Here's how the part is built. I have some questions about the finished solid (model axes, mm). Face numbers are marked on the shaded views. A direction names the side the tool comes from. Round coordinates to 2 decimals unless told otherwise and drop trailing zeros. Loops run counter-clockwise (first coordinate to the right, second up) from the corner with the lowest first, then second, coordinate; pieces in that order, holes last. Notation, with made-up numbers: M 47,38 L 51,38 A27 ccw 51,68 Z; hole C 61.25,46.25 d7. An arc over 180 degrees is marked long. Use a Markdown table: item, result.
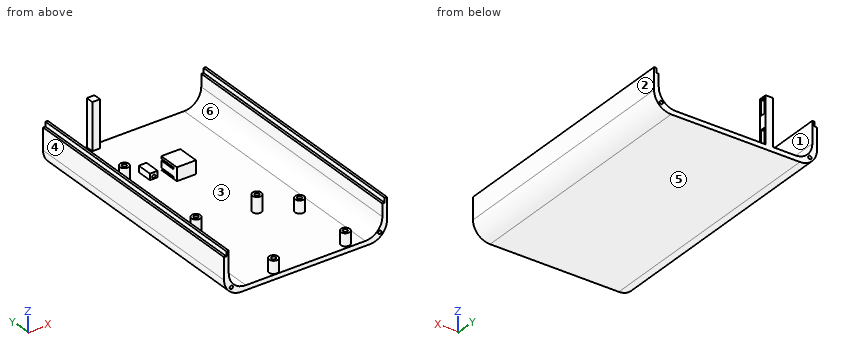
from build123d import *

# Parameters (mm, degrees)
EXTRUDE_1_DEPTH       = 162.5
SKETCH_2_W            = 1.5
SKETCH_2_H            = 162.5
EXTRUDE_2_DEPTH       = 3
SKETCH_2_4_W          = 1.5
SKETCH_2_4_H          = 162.5
CUT_EXTRUDE_2_DEPTH   = 3
SKETCH_3_R            = 1.05
CUT_EXTRUDE_3_DEPTH   = 4
CUT_EXTRUDE_START     = -4
SKETCH_4_R            = 1.05
CUT_EXTRUDE_4_DEPTH   = 4
SKETCH_6_R            = 2.9
SKETCH_6_R_2          = 1.4
EXTRUDE_1_2_DEPTH     = 10
SKETCH_7_R            = 2.9
SKETCH_7_R_2          = 1.4
EXTRUDE_2_2_DEPTH     = 8
EXTRUDE_4_DEPTH       = 8.5
CUT_EXTRUDE_6_REACH   = 176.56
SKETCH_13_W           = 1.2
SKETCH_13_H           = 11
EXTRUDE_START         = 1.4
EXTRUDE_5_OUTLINE_W   = 0.5
EXTRUDE_5_OUTLINE_H   = 1.8
EXTRUDE_5_DEPTH       = 4.4
EXTRUDE_5_2_OUTLINE_W = 5
EXTRUDE_5_2_OUTLINE_H = 10
EXTRUDE_5_2_DEPTH     = 4
EXTRUDE_START_2       = 116
EXTRUDE_6_OUTLINE_R   = 1.05
EXTRUDE_6_DEPTH       = 10
EXTRUDE_START_3       = 157.5
EXTRUDE_6_2_OUTLINE_W = 5
EXTRUDE_6_2_OUTLINE_H = 30
EXTRUDE_6_2_DEPTH     = 5
EXTRUDE_START_4       = -7.5
EXTRUDE_7_OUTLINE_W   = 2.9
EXTRUDE_7_OUTLINE_H   = 2.85
EXTRUDE_7_DEPTH       = 9.65
EXTRUDE_START_5       = 10.85
EXTRUDE_7_2_OUTLINE_W = 2.9
EXTRUDE_7_2_OUTLINE_H = 2.85
EXTRUDE_7_2_DEPTH     = 9.65
EXTRUDE_START_6       = -1.5
EXTRUDE_7_3_OUTLINE_W = 8.3
EXTRUDE_7_3_OUTLINE_H = 11.95
EXTRUDE_7_3_DEPTH     = 1.5


# Read off the part's stored shape, not the designer's step: 凸台-拉伸5, 凸台-拉伸6, 凸台-拉伸7
with BuildPart() as part:
    # 草图1 → Extrude 1 (new body)
    with BuildSketch(Plane(origin=(0, 0, 0), x_dir=(1, 0, 0), z_dir=(0, 1, 0))):
        with BuildLine():
            Line((-3, 0), (-3, 14))
            ThreePointArc((-3, 14), (0.221825407, 21.778174593), (8, 25))
            Line((8, 25), (91, 25))
            ThreePointArc((91, 25), (98.778174593, 21.778174593), (102, 14))
            Line((102, 14), (102, 0))
            Line((102, 0), (99, 0))
            Line((99, 0), (99, 11))
            ThreePointArc((99, 11), (95.778174593, 18.778174593), (88, 22))
            Line((88, 22), (11, 22))
            ThreePointArc((11, 22), (3.221825407, 18.778174593), (0, 11))
            Line((0, 11), (0, 0))
            Line((0, 0), (-3, 0))
        make_face()
    extrude(amount=EXTRUDE_1_DEPTH)

    # 草图2 → Extrude 2 (add)
    with BuildSketch(Plane.XY):
        with Locations((-0.75, 81.25)):
            Rectangle(SKETCH_2_W, SKETCH_2_H)
    extrude(amount=EXTRUDE_2_DEPTH)

    # 草图2<4> → 切除-拉伸2 (cut)
    with BuildSketch(Plane.XY):
        with Locations((99.75, 81.25)):
            Rectangle(SKETCH_2_4_W, SKETCH_2_4_H)
    extrude(amount=-CUT_EXTRUDE_2_DEPTH, mode=Mode.SUBTRACT)

    # 草图3 → 切除-拉伸3 (cut)
    with BuildSketch(Plane(origin=(0, 162.5, 0), x_dir=(1, 0, 0), z_dir=(0, 1, 0))):
        with Locations(Location((1.61916848, 20, 0), (0, 0, 270))):
            Circle(SKETCH_3_R)
        with Locations(Location((97.38083152, 20, 0), (0, 0, 270))):
            Circle(SKETCH_3_R)
    extrude(amount=-CUT_EXTRUDE_3_DEPTH, mode=Mode.SUBTRACT)

    # 草图4 → 切除-拉伸4 (cut)
    with BuildSketch(Plane.XZ.offset(CUT_EXTRUDE_START)):
        with Locations(Location((1.61916848, -20, 0), (0, 0, 90))):
            Circle(SKETCH_4_R)
        with Locations(Location((97.38083152, -20, 0), (0, 0, 90))):
            Circle(SKETCH_4_R)
    extrude(amount=CUT_EXTRUDE_4_DEPTH, mode=Mode.SUBTRACT)

    # 草图6 → Extrude 1 2 (add)
    # profile 1 of 3: a face of its own
    with BuildSketch(Plane.XY.offset(-22)):
        with Locations((20.69, 122.5)):
            Circle(SKETCH_6_R)
        with Locations((20.69, 122.5)):
            Circle(SKETCH_6_R_2, mode=Mode.SUBTRACT)
    # profile 2 of 3: a face of its own
    with BuildSketch(Plane.XY.offset(-22)):
        with Locations((20.69, 58.19)):
            Circle(SKETCH_6_R)
        with Locations((20.69, 58.19)):
            Circle(SKETCH_6_R_2, mode=Mode.SUBTRACT)
    # profile 3 of 3: a face of its own
    with BuildSketch(Plane.XY.offset(-22)):
        with Locations((60, 58.19)):
            Circle(SKETCH_6_R)
        with Locations((60, 58.19)):
            Circle(SKETCH_6_R_2, mode=Mode.SUBTRACT)
    extrude(amount=EXTRUDE_1_2_DEPTH)

    # 草图7 → Extrude 2 2 (add)
    # profile 1 of 3: a face of its own
    with BuildSketch(Plane.XY.offset(-22)):
        with Locations((78, 4)):
            Circle(SKETCH_7_R)
        with Locations((78, 4)):
            Circle(SKETCH_7_R_2, mode=Mode.SUBTRACT)
    # profile 2 of 3: a face of its own
    with BuildSketch(Plane.XY.offset(-22)):
        with Locations((31.2, 3.2)):
            Circle(SKETCH_7_R)
        with Locations((31.2, 3.2)):
            Circle(SKETCH_7_R_2, mode=Mode.SUBTRACT)
    # profile 3 of 3: a face of its own
    with BuildSketch(Plane.XY.offset(-22)):
        with Locations((78, 45)):
            Circle(SKETCH_7_R)
        with Locations((78, 45)):
            Circle(SKETCH_7_R_2, mode=Mode.SUBTRACT)
    extrude(amount=EXTRUDE_2_2_DEPTH)

    # 草图12 → 凸台-拉伸4 (add)
    with BuildSketch(Plane.XY.offset(-22)):
        Polygon((45.35, 120.9), (45.35, 108.95), (53.65, 108.95), (53.65, 120.9), (55.65, 120.9), (55.65, 106.9), (43.35, 106.9), (43.35, 120.9), align=None)
    extrude(amount=EXTRUDE_4_DEPTH)

    # 切除-拉伸6: up to this face of the body (flat: up to its plane)
    cut_extrude_6_end = Plane(part.part.faces().sort_by_distance((43.35, 113.9, -17.75))[0])
    # 草图13 → 切除-拉伸6 (cut, up to the picked face)
    with BuildSketch(Plane(origin=(55.65, 0, 0), x_dir=(0, 0, -1), z_dir=(1, 0, 0)), mode=Mode.PRIVATE) as cut_extrude_6_sk1:
        with Locations((15.6, 115.4)):
            Rectangle(SKETCH_13_W, SKETCH_13_H)
    cut_extrude_6_tool1 = split(extrude(cut_extrude_6_sk1.sketch, amount=-CUT_EXTRUDE_6_REACH, mode=Mode.PRIVATE), bisect_by=cut_extrude_6_end, keep=Keep.BOTH, mode=Mode.PRIVATE)
    # 草图13 → 切除-拉伸6 (cut, up to the picked face)
    with BuildSketch(Plane(origin=(55.65, 0, 0), x_dir=(0, 0, -1), z_dir=(1, 0, 0)), mode=Mode.PRIVATE) as cut_extrude_6_sk2:
        with Locations((21.2, 115.4)):
            Rectangle(SKETCH_13_W, SKETCH_13_H)
    cut_extrude_6_tool2 = split(extrude(cut_extrude_6_sk2.sketch, amount=-CUT_EXTRUDE_6_REACH, mode=Mode.PRIVATE), bisect_by=cut_extrude_6_end, keep=Keep.BOTH, mode=Mode.PRIVATE)
    add(cut_extrude_6_tool1.solids().sort_by(Axis((55.65, 115.4, -15.6), (-1, 0, 0)))[0], mode=Mode.SUBTRACT)
    add(cut_extrude_6_tool2.solids().sort_by(Axis((55.65, 115.4, -21.2), (-1, 0, 0)))[0], mode=Mode.SUBTRACT)

    # 凸台-拉伸5 outline → 凸台-拉伸5 (cut)
    with BuildSketch(Plane.XY.offset(-22).offset(EXTRUDE_START)):
        with Locations((53.9, 118.25)):
            Rectangle(EXTRUDE_5_OUTLINE_W, EXTRUDE_5_OUTLINE_H)
        with Locations((45.1, 118.25)):
            Rectangle(EXTRUDE_5_OUTLINE_W, EXTRUDE_5_OUTLINE_H)
    extrude(amount=EXTRUDE_5_DEPTH, mode=Mode.SUBTRACT)

    # Extrude 5 2 outline → Extrude 5 2 (add)
    with BuildSketch(Plane.XY.offset(-22)):
        with Locations((35, 121)):
            Rectangle(EXTRUDE_5_2_OUTLINE_W, EXTRUDE_5_2_OUTLINE_H)
    extrude(amount=EXTRUDE_5_2_DEPTH)

    # 凸台-拉伸6 outline → 凸台-拉伸6 (cut)
    with BuildSketch(Plane(origin=(0, 0, 0), x_dir=(1, 0, 0), z_dir=(0, 1, 0)).offset(EXTRUDE_START_2)):
        with Locations((35, 20.5)):
            Circle(EXTRUDE_6_OUTLINE_R)
    extrude(amount=EXTRUDE_6_DEPTH, mode=Mode.SUBTRACT)

    # Extrude 6 2 outline → Extrude 6 2 (add)
    with BuildSketch(Plane(origin=(0, 0, 0), x_dir=(1, 0, 0), z_dir=(0, 1, 0)).offset(EXTRUDE_START_3)):
        with Locations((27.7, 7)):
            Rectangle(EXTRUDE_6_2_OUTLINE_W, EXTRUDE_6_2_OUTLINE_H)
    extrude(amount=EXTRUDE_6_2_DEPTH)

    # 凸台-拉伸7 outline → 凸台-拉伸7 (cut)
    with BuildSketch(Plane.XY.offset(-13.5).offset(EXTRUDE_START_4)):
        with Locations((28.75, 160.075)):
            Rectangle(EXTRUDE_7_OUTLINE_W, EXTRUDE_7_OUTLINE_H)
    extrude(amount=EXTRUDE_7_DEPTH, mode=Mode.SUBTRACT)

    # Extrude 7 2 outline → Extrude 7 2 (cut)
    with BuildSketch(Plane.XY.offset(-13.5).offset(EXTRUDE_START_5)):
        with Locations((28.75, 160.075)):
            Rectangle(EXTRUDE_7_2_OUTLINE_W, EXTRUDE_7_2_OUTLINE_H)
    extrude(amount=EXTRUDE_7_2_DEPTH, mode=Mode.SUBTRACT)

    # Extrude 7 3 outline → Extrude 7 3 (add)
    with BuildSketch(Plane.XY.offset(-13.5).offset(EXTRUDE_START_6)):
        with Locations((49.5, 114.925)):
            Rectangle(EXTRUDE_7_3_OUTLINE_W, EXTRUDE_7_3_OUTLINE_H)
    extrude(amount=EXTRUDE_7_3_DEPTH)


solid = part.part
1. Imagine slicing it at C-C, the plane x = 72. Write out the boundary of the cut face in (y, z).
Answer sheet:
| item | result |
|---|---|
| outline | M 0,-25 L 162.5,-25 L 162.5,-22 L 0,-22 Z |
2. We'd pull the mould along X, two halves only. Please class the marked faces 1, 2, 3 and 4: +X half, -X half, draft (parallel to the pull), parting line (faces both ways), or undercut.
Answer sheet:
| item | result |
|---|---|
| face 1 | undercut |
| face 2 | +X half |
| face 3 | undercut |
| face 4 | -X half |
3. Which directions (+Z, -Z, +X, -X, +Y, -Y) give clear straight access to the entire face, cutting with the end or side of a thin tool? Please do the marked faces 5 and 6.
Answer sheet:
| item | result |
|---|---|
| face 5 | -Z, +X, -X, +Y, -Y |
| face 6 | +Z, +Y, -Y |
4. Imagine slicing it at D-D, the plane x = 93.5. Write out the boundary of the cut face in (y, z), then the cut area to 3 significant figures.
Answer sheet:
| item | result |
|---|---|
| outline | M 0,-24.71 L 162.5,-24.71 L 162.5,-20.53 L 0,-20.53 Z |
| area | 680 mm2 |
5. Imagine slicing it at B-B, the plane y = 74. Write out the boundary of the cut face in (x, z).
Answer sheet:
| item | result |
|---|---|
| outline | M -3,-14 A11 ccw 8,-25 L 91,-25 A11 ccw 102,-14 L 102,0 L 100.5,0 L 100.5,-3 L 99,-3 L 99,-11 A11 cw 88,-22 L 11,-22 A11 cw 0,-11 L 0,3 L -1.5,3 L -1.5,0 L -3,0 Z |
6. I need wall thicknesses on probe 1 along Y at (x, z) = (78, -19.5); probe 2 along X at (y, z) = (71, -6); probe 3 along Y at (x, z) = (21.5, -15.5). Which ranges of each line are inside material? Lowest first, please. Write a range as from..to.
Answer sheet:
| item | result |
|---|---|
| probe 1 | 1.1..2.6, 5.4..6.9, 42.1..43.6, 46.4..47.9 |
| probe 2 | -3..0, 99..102 |
| probe 3 | 55.41..57.05, 59.33..60.97, 119.72..121.36, 123.64..125.28 |
7. For pin 1 Ø1 at (x, z) = (44.5, -19) entering from +Y; pin 2 Ø1.5 at (x, z) = (27, -1.5) entering from -Y; pin 3 Ø1.4 at (y, z) = (118, -18.5) entering from +X, each with a flat end and sliding along its axis, tell me the tip position at first contact or that it passes through.
Answer sheet:
| item | result |
|---|---|
| pin 1 | y = 120.9 |
| pin 2 | y = 157.5 |
| pin 3 | x = 101.32 |
8. Imagine slicing it at A-A, the plane z = -6. Write out the boundary of the cut face in (x, y).
Answer sheet:
| item | result |
|---|---|
| outline | M -3,0 L 0,0 L 0,162.5 L -3,162.5 Z; M 25.2,157.5 L 30.2,157.5 L 30.2,162.5 L 25.2,162.5 Z; M 99,0 L 102,0 L 102,162.5 L 99,162.5 Z |
